Model file for the job. Use its own axes, mm. A direction names the side the tool comes from. Round coordinates to 2 decimals unless told otherwise and drop trailing zeros. Loops run counter-clockwise (first coordinate to the right, second up) from the corner with the lowest first, then second, coordinate; pieces in that order, holes last. Notation, with made-up numbers: (13, 43) - (54, 43) arc R27 cw to (54, 74) - close; hole circle Ø5 at (16.5, -13.75). An arc over 180 degrees is marked (long way). Answer as a JSON object with one key per item and string values.
from build123d import *

# Parameters (mm, degrees)
F0_R     = 50.421677
F1_DEPTH = 150
F2_SIZE  = 5
F3_R     = 10.184595
F4_DEPTH = 16
F5_SIZE  = 5
F6_R     = 10.343213
F7_DEPTH = 16


with BuildPart() as f1:
    # F0 (on Front) → F1 (new body)
    with BuildSketch(Plane.XZ):
        Circle(F0_R)
    extrude(amount=F1_DEPTH)

    # F2
    f2_edges = [f1.edges().sort_by_distance(p)[0] for p in [
        (-50.421677, -150, 0),
    ]]
    chamfer(f2_edges, length=F2_SIZE)

    # F3 (on face) → F4 (join)
    with BuildSketch(Plane.XZ.offset(150)):
        Circle(F3_R)
    extrude(amount=F4_DEPTH)

    # F5
    f5_edges = [f1.edges().sort_by_distance(p)[0] for p in [
        (-50.421677, 0, 0),
    ]]
    chamfer(f5_edges, length=F5_SIZE)

    # F6 (on face) → F7 (join)
    with BuildSketch(Plane(origin=(0, 0, 0), x_dir=(-1, 0, 0), z_dir=(0, 1, 0))):
        Circle(F6_R)
    extrude(amount=F7_DEPTH)


solid = f1.part
1) Drop flat-ended pins along their axis: P1, Ø10, axis at x = -24.5, y = -124.5, coming from the +Z side; P2, Ø6, axis at y = -28, z = -7.5, coming from the +X side; P3, Ø10, axis at y = -74.5, z = 23.5, coming from the +X side. Give the stop position or say it passes through.
Values follow:
{"P1": "z = 46.5", "P2": "x = 50.22", "P3": "x = 46.91"}
2) Tool access for faces 1 (the cylindrical face through (-2.21, -157.89, -9.94)), 2 (the cylindrical face through (-5.56, 7.89, 8.72)), 3 (the flat face through (0, -166, 0)): list every direction of +Z, -Z, +X, -X, +Y, -Y with a clear straight run to the whole face (end or side of a thin tool).
Values follow:
{"face 1": "-Y", "face 2": "+Y", "face 3": "+Z, -Z, +X, -X, -Y"}
3) Slice it at C-C on y = -142. List the corners of the cut face in (x, z), then the cut area to 3 significant figures.
Values follow:
{"outline": "circle Ø100.84 at (0, 0)", "area": "7,990 mm²"}
4) Slice it at B-B on x = 0. List the corners of the cut face in (y, z).
Values follow:
{"outline": "(-166, -10.18) - (-150, -10.18) - (-150, -45.42) - (-145, -50.42) - (-5, -50.42) - (0, -45.42) - (0, -10.34) - (16, -10.34) - (16, 10.34) - (0, 10.34) - (0, 45.42) - (-5, 50.42) - (-145, 50.42) - (-150, 45.42) - (-150, 10.18) - (-166, 10.18) - close"}
5) Slice it at A-A on z = 0. List the corners of the cut face in (x, y), then the cut area to 3 significant figures.
Values follow:
{"outline": "(-50.42, -145) - (-45.42, -150) - (-10.18, -150) - (-10.18, -166) - (10.18, -166) - (10.18, -150) - (45.42, -150) - (50.42, -145) - (50.42, -5) - (45.42, 0) - (10.34, 0) - (10.34, 16) - (-10.34, 16) - (-10.34, 0) - (-45.42, 0) - (-50.42, -5) - close", "area": "15,700 mm²"}
6) Probe probe 1 along Y at (x, z) = (22, -28); probe 2 along Z at (x, y) = (2, -55.5); probe 3 along X at (y, z) = (-65, 43). List the from-to ranges inside material, lowest first.
Values follow:
{"probe 1": "-150 to 0", "probe 2": "-50.38 to 50.38", "probe 3": "-26.33 to 26.33"}
